Can you work these out from the model? Positions are in its coordinate system, mm. A direction names the side the tool comes from. Round coordinates to 2 decimals unless told otherwise and drop trailing zeros. Write each loop counter-clockwise with the first axis right and the second up, starting at its lowest first coordinate (ties: lowest second). Pieces come first, ordered by that corner, then holes. Notation, with made-up numbers: M 61,-24.75 L 73,-24.75 A13 cw 73,-11.75 Z; hole C 79.5,59.5 d2. An arc over 180 degrees is marked long. Answer in a Markdown table with one row per item. Add a question column.
(1) Suppose I cut it at C-C, the plane x = 5.5. Write out the boundary of the cut face in (y, z), then the cut area to 3 significant figures.
(2) If we mould it in two halves opening along Y, with no side actions, what happens to faces 3 (the face through (-2, 2, 2)), 4 (the face through (18.31, 2, 2)), 5 (the face through (-2, -18.063, 2))? For each: released by +Y, released by -Y, zero draft, split by the parting line, or undercut.
(3) I'm going to push a flat-ended pin straight in: pin 1 (5 mm diameter, centred on x = -7, y = -9.5, fed in from +Z). Where does the tip first touch, or does it pass through?
(4) Suppose I cut it at B-B, the plane y = 0. Write out the boundary of the cut face in (x, z).
(5) Suppose I cut it at A-A, the plane z = 3.05. Write out the boundary of the cut face in (x, y), then the cut area to 3 significant figures.
(6) If I drill on probe 1 along Y at (x, z) = (-15, 2.1); probe 2 along X at (y, z) = (-6.5, 3.05); probe 3 along Z at (x, y) = (-14.5, -6.5), over which ranges is the centre line in solid material (lowest first)?
(7) For faces 1 (the face through (16.31, 2, 3)), 2 (the face through (-21.69, 2, 2)), which set-ups out of +Z, -Z, +X, -X, +Y, -Y let a thin tool reach every point of the face, with its end or its side?
from build123d import *

# Parameters (mm, degrees)
F0_W     = 40
F0_H     = 40
F1_DEPTH = 4
F2_W     = 36.000001
F2_H     = 36.000001
F3_DEPTH = 2
F4_W     = 36
F4_H     = 36
F5_DEPTH = 2


with BuildPart() as f1:
    # F0 (on Top) → F1 (new body)
    with BuildSketch(Plane.XY):
        with Locations((-1.689615, 1.937058)):
            Rectangle(F0_W, F0_H)
    extrude(amount=F1_DEPTH)

    # F2 (on face) → F3 (join)
    with BuildSketch(Plane.XY.offset(4)):
        with Locations((-1.689615, 1.937058)):
            Rectangle(F2_W, F2_H)
    extrude(amount=-F3_DEPTH)

    # F4 (on face) → F5 (cut)
    with BuildSketch(Plane.XY.offset(4)):
        with Locations((-1.689615, 1.937058)):
            Rectangle(F4_W, F4_H)
    extrude(amount=-F5_DEPTH, mode=Mode.SUBTRACT)


solid = f1.part
Calculated:
| question | item | result |
|---|---|---|
| 1 | outline | M -18.06,0 L 21.94,0 L 21.94,4 L 19.94,4 L 19.94,2 L -16.06,2 L -16.06,4 L -18.06,4 Z |
| 1 | area | 88.0 mm² |
| 2 | face 3 | undercut |
| 2 | face 4 | zero draft |
| 2 | face 5 | released by -Y |
| 3 | pin 1 | z = 2 |
| 4 | outline | M -21.69,0 L 18.31,0 L 18.31,4 L 16.31,4 L 16.31,2 L -19.69,2 L -19.69,4 L -21.69,4 Z |
| 5 | outline | M -21.69,-18.06 L 18.31,-18.06 L 18.31,21.94 L -21.69,21.94 Z; hole M -19.69,-16.06 L 16.31,-16.06 L 16.31,19.94 L -19.69,19.94 Z |
| 5 | area | 304 mm² |
| 6 | probe 1 | -18.06 to -16.06, 19.94 to 21.94 |
| 6 | probe 2 | -21.69 to -19.69, 16.31 to 18.31 |
| 6 | probe 3 | 0 to 2 |
| 7 | face 1 | +Z |
| 7 | face 2 | +Z, -Z, -X, +Y, -Y |
